Geometry check sheet. Reference: the model listing, model coordinates, mm. Face numbers are marked on the shaded views. Give positions to 0.01 mm unless a question says otherwise; leave off trailing zeros. Loops run counter-clockwise (first coordinate to the right, second up) from the corner with the lowest first, then second, coordinate; pieces in that order, holes last. Notation, with made-up numbers: (55.25, 25) -> (101.25, 25) arc R26 ccw to (101.25, 39) -> close; hole circle Ø8 at (-17.75, 36.25). An arc over 180 degrees is marked (long way). One line per item, written item: value. Start each with the question number.
(1) Sectioned sample at B-B, the plane z = 0. Record the cut outline in (x, y).
(2) Draft check along Z on the marked faces 1, 2 and 3. Enter one of: pulls with the +Z half, pulls with the -Z half, needs draft (parallel to the pull), parting line crosses it, or undercut.
(3) Sectioned sample at C-C, the plane y = 83.5. Record the cut outline in (x, z), then the cut area to 3 significant figures.
(4) Gauge pin test, flat ends, axial feed: pin 1 Ø7 at (y, z) = (90, 0) entering from -X; pin 2 Ø1 at (y, z) = (58.5, 8) entering from +X; pin 3 Ø1 at (x, z) = (-8, -2) entering from +Y; pin 4 Ø1.5 at (x, y) = (2.5, 21) entering from +Z. Record the tip position at first contact, or that the pin passes through.
(5) Sectioned sample at A-A, the plane y = 9.5. Record the cut outline in (x, z).
(6) Scan lines: line 1 along Y through (x, z) = (-1.5, 0); line 2 along X through (y, z) = (49.5, 0); line 3 along Y through (x, z) = (0.75, -6.5). Record each from-to range of solid material in increasing order. Write a range as from..to.
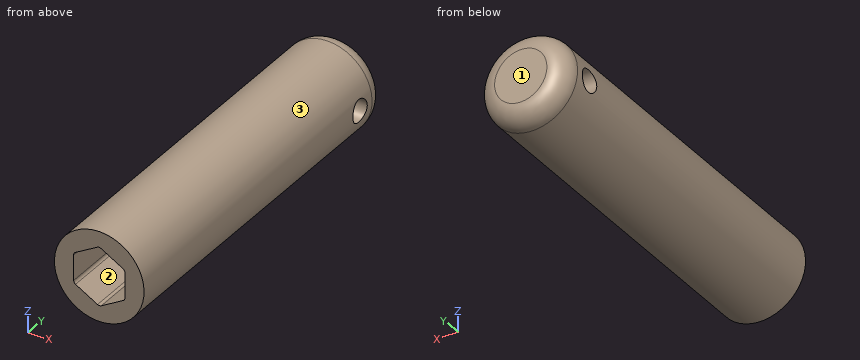
from build123d import *

# Parameters (mm, degrees)
SKETCH_1_R          = 12
SKETCH_1_R_2        = 6
EXTRUDE_1_DEPTH     = 80
CUT_EXTRUDE_1_DEPTH = 17
FILLET_1_R          = 1
SKETCH_3_R          = 12
EXTRUDE_2_DEPTH     = 20
FILLET_2_R          = 5
SKETCH_4_R          = 3
CUT_EXTRUDE_3_DEPTH = 22.5


with BuildPart() as part:
    # Эскиз1 → Вытянуть1 (new body)
    with BuildSketch(Plane(origin=(0, 0, 0), x_dir=(1, 0, 0), z_dir=(0, 1, 0))):
        with Locations(Location((0, 0, 0), (0, 0, 270))):
            Circle(SKETCH_1_R)
        with Locations(Location((0, 0, 0), (0, 0, 270))):
            Circle(SKETCH_1_R_2, mode=Mode.SUBTRACT)
    extrude(amount=EXTRUDE_1_DEPTH)

    # Эскиз2 → Вырез-Вытянуть1 (cut)
    with BuildSketch(Plane.XZ):
        Polygon((6.883625854, -3.933459236), (6.84828855, 3.994665242), (-0.035337304, 7.928124478), (-6.883625854, 3.933459236), (-6.84828855, -3.994665242), (0.035337304, -7.928124478), align=None)
    extrude(amount=-CUT_EXTRUDE_1_DEPTH, mode=Mode.SUBTRACT)

    # Скругление1
    fillet_1_edges = [part.edges().sort_by_distance(p)[0] for p in [
        (6.883625854, 8.5, -3.933459236),
        (0.035337304, 8.5, -7.928124478),
        (-6.84828855, 8.5, -3.994665242),
        (-6.883625854, 8.5, 3.933459236),
        (-0.035337304, 8.5, 7.928124478),
        (6.84828855, 8.5, 3.994665242),
    ]]
    fillet(fillet_1_edges, radius=FILLET_1_R)

    # Эскиз3 → Вытянуть2 (add)
    with BuildSketch(Plane(origin=(0, 80, 0), x_dir=(1, 0, 0), z_dir=(0, 1, 0))):
        with Locations(Location((0, 0, 0), (0, 0, 270))):
            Circle(SKETCH_3_R)
    extrude(amount=EXTRUDE_2_DEPTH)

    # Скругление2
    fillet_2_edges = [part.edges().sort_by_distance(p)[0] for p in [
        (0, 100, -12),
    ]]
    fillet(fillet_2_edges, radius=FILLET_2_R)

    # Эскиз4 → Вытянуть3 (cut, symmetric)
    with BuildSketch(Plane(origin=(0, 0, 0), x_dir=(0, 0, -1), z_dir=(1, 0, 0))):
        with Locations((0, 90)):
            Circle(SKETCH_4_R)
    extrude(amount=CUT_EXTRUDE_3_DEPTH, both=True, mode=Mode.SUBTRACT)


solid = part.part
Calculated:
1. outline: (-12, 0) -> (-6.87, 0) -> (-6.87, 17) -> (-6, 17) -> (-6, 80) -> (6, 80) -> (6, 17) -> (6.87, 17) -> (6.87, 0) -> (12, 0) -> (12, 87) -> (-12, 87) -> close; (-12, 93) -> (12, 93) -> (12, 95) arc R5 ccw to (7, 100) -> (-7, 100) arc R5 ccw to (-12, 95) -> close
2. face 1: needs draft
2. face 2: undercut
2. face 3: parting line crosses it
3. outline: circle Ø24 at (0, 0)
3. area: 452 mm2
4. pin 1: stops at x = -12
4. pin 2: stops at x = 9.37
4. pin 3: stops at y = 99.94
4. pin 4: stops at z = 11.87
5. outline: circle Ø24 at (0, 0); hole (-6.88, 3.36) -> (-6.85, -3.42) arc R1 ccw to (-6.35, -4.28) -> (-0.47, -7.64) arc R1 ccw to (0.53, -7.64) -> (6.38, -4.22) arc R1 ccw to (6.88, -3.36) -> (6.85, 3.42) arc R1 ccw to (6.35, 4.28) -> (0.47, 7.64) arc R1 ccw to (-0.53, 7.64) -> (-6.38, 4.22) arc R1 ccw to start
6. line 1: y = 80..87, 93..100
6. line 2: x = -12..-6, 6..12
6. line 3: y = 17..100
